from build123d import *

# Parameters (mm, degrees)
F2_DEPTH = 25
F3_DEPTH = 25


with BuildPart() as f2:
    # F1 (on Front) → F2 (new body)
    with BuildSketch(Plane.XZ):
        with BuildLine():
            ThreePointArc((14.696938, -3), (14.924042, -1.507634), (15, 0))
            ThreePointArc((15, 0), (14.924042, 1.507634), (14.696938, 3))
            ThreePointArc((14.696938, 3), (13.858193, 5.740251), (12.513625, 8.270985))
            ThreePointArc((12.513625, 8.270985), (10.606602, 10.606602), (8.270985, 12.513625))
            ThreePointArc((8.270985, 12.513625), (5.740251, 13.858193), (3, 14.696938))
            ThreePointArc((3, 14.696938), (0, 15), (-3, 14.696938))
            ThreePointArc((-3, 14.696938), (-5.740251, 13.858193), (-8.270985, 12.513625))
            ThreePointArc((-8.270985, 12.513625), (-10.606602, 10.606602), (-12.513625, 8.270985))
            ThreePointArc((-12.513625, 8.270985), (-13.858193, 5.740251), (-14.696938, 3))
            ThreePointArc((-14.696938, 3), (-15, 0), (-14.696938, -3))
            ThreePointArc((-14.696938, -3), (-13.858193, -5.740251), (-12.513625, -8.270985))
            ThreePointArc((-12.513625, -8.270985), (-10.606602, -10.606602), (-8.270985, -12.513625))
            ThreePointArc((-8.270985, -12.513625), (-5.740251, -13.858193), (-3, -14.696938))
            ThreePointArc((-3, -14.696938), (0, -15), (3, -14.696938))
            ThreePointArc((3, -14.696938), (5.740251, -13.858193), (8.270985, -12.513625))
            ThreePointArc((8.270985, -12.513625), (10.606602, -10.606602), (12.513625, -8.270985))
            ThreePointArc((12.513625, -8.270985), (13.858193, -5.740251), (14.696938, -3))
        make_face()
        with BuildLine():
            ThreePointArc((-12.513625, 8.270985), (-10.606602, 10.606602), (-8.270985, 12.513625))
            Line((-8.270985, 12.513625), (-11.860811, 16.103452))
            ThreePointArc((-11.860811, 16.103452), (-14.142136, 14.142136), (-16.103452, 11.860811))
            Line((-16.103452, 11.860811), (-12.513625, 8.270985))
        make_face()
        with BuildLine():
            ThreePointArc((-14.696938, -3), (-15, 0), (-14.696938, 3))
            Line((-14.696938, 3), (-19.77372, 3))
            ThreePointArc((-19.77372, 3), (-20, 0), (-19.77372, -3))
            Line((-19.77372, -3), (-14.696938, -3))
        make_face()
        with BuildLine():
            Line((-11.860811, -16.103452), (-8.270985, -12.513625))
            ThreePointArc((-8.270985, -12.513625), (-10.606602, -10.606602), (-12.513625, -8.270985))
            Line((-12.513625, -8.270985), (-16.103452, -11.860811))
            ThreePointArc((-16.103452, -11.860811), (-14.142136, -14.142136), (-11.860811, -16.103452))
        make_face()
        with BuildLine():
            Line((3, -19.77372), (3, -14.696938))
            ThreePointArc((3, -14.696938), (0, -15), (-3, -14.696938))
            Line((-3, -14.696938), (-3, -19.77372))
            ThreePointArc((-3, -19.77372), (0, -20), (3, -19.77372))
        make_face()
        with BuildLine():
            Line((16.103452, -11.860811), (12.513625, -8.270985))
            ThreePointArc((12.513625, -8.270985), (10.606602, -10.606602), (8.270985, -12.513625))
            Line((8.270985, -12.513625), (11.860811, -16.103452))
            ThreePointArc((11.860811, -16.103452), (14.142136, -14.142136), (16.103452, -11.860811))
        make_face()
        with BuildLine():
            ThreePointArc((14.696938, 3), (14.924042, 1.507634), (15, 0))
            ThreePointArc((15, 0), (14.924042, -1.507634), (14.696938, -3))
            Line((14.696938, -3), (19.77372, -3))
            ThreePointArc((19.77372, -3), (20, 0), (19.77372, 3))
            Line((19.77372, 3), (14.696938, 3))
        make_face()
        with BuildLine():
            ThreePointArc((8.270985, 12.513625), (10.606602, 10.606602), (12.513625, 8.270985))
            Line((12.513625, 8.270985), (16.103452, 11.860811))
            ThreePointArc((16.103452, 11.860811), (14.142136, 14.142136), (11.860811, 16.103452))
            Line((11.860811, 16.103452), (8.270985, 12.513625))
        make_face()
        with BuildLine():
            ThreePointArc((-3, 14.696938), (0, 15), (3, 14.696938))
            Line((3, 14.696938), (3, 19.77372))
            ThreePointArc((3, 19.77372), (0, 20), (-3, 19.77372))
            Line((-3, 19.77372), (-3, 14.696938))
        make_face()
    extrude(amount=F2_DEPTH)

    # F0 (on Front) → F3 (cut)
    with BuildSketch(Plane.XZ):
        with BuildLine():
            Line((-5.338161, 7.245967), (-4.582543, 5.937197))
            ThreePointArc((-4.582543, 5.937197), (-5.303301, 5.303301), (-5.937197, 4.582543))
            Line((-5.937197, 4.582543), (-7.245967, 5.338161))
            ThreePointArc((-7.245967, 5.338161), (-7.794229, 4.5), (-8.245967, 3.606111))
            Line((-8.245967, 3.606111), (-6.937197, 2.850492))
            ThreePointArc((-6.937197, 2.850492), (-7.244444, 1.941143), (-7.433034, 1))
            Line((-7.433034, 1), (-8.944272, 1))
            ThreePointArc((-8.944272, 1), (-9, 0), (-8.944272, -1))
            Line((-8.944272, -1), (-7.433034, -1))
            ThreePointArc((-7.433034, -1), (-7.244444, -1.941143), (-6.937197, -2.850492))
            Line((-6.937197, -2.850492), (-8.245967, -3.606111))
            ThreePointArc((-8.245967, -3.606111), (-7.794229, -4.5), (-7.245967, -5.338161))
            Line((-7.245967, -5.338161), (-5.937197, -4.582543))
            ThreePointArc((-5.937197, -4.582543), (-5.303301, -5.303301), (-4.582543, -5.937197))
            Line((-4.582543, -5.937197), (-5.338161, -7.245967))
            ThreePointArc((-5.338161, -7.245967), (-4.5, -7.794229), (-3.606111, -8.245967))
            Line((-3.606111, -8.245967), (-2.850492, -6.937197))
            ThreePointArc((-2.850492, -6.937197), (-1.941143, -7.244444), (-1, -7.433034))
            Line((-1, -7.433034), (-1, -8.944272))
            ThreePointArc((-1, -8.944272), (0, -9), (1, -8.944272))
            Line((1, -8.944272), (1, -7.433034))
            ThreePointArc((1, -7.433034), (1.941143, -7.244444), (2.850492, -6.937197))
            Line((2.850492, -6.937197), (3.606111, -8.245967))
            ThreePointArc((3.606111, -8.245967), (4.5, -7.794229), (5.338161, -7.245967))
            Line((5.338161, -7.245967), (4.582543, -5.937197))
            ThreePointArc((4.582543, -5.937197), (5.303301, -5.303301), (5.937197, -4.582543))
            Line((5.937197, -4.582543), (7.245967, -5.338161))
            ThreePointArc((7.245967, -5.338161), (7.794229, -4.5), (8.245967, -3.606111))
            Line((8.245967, -3.606111), (6.937197, -2.850492))
            ThreePointArc((6.937197, -2.850492), (7.244444, -1.941143), (7.433034, -1))
            Line((7.433034, -1), (8.944272, -1))
            ThreePointArc((8.944272, -1), (9, 0), (8.944272, 1))
            Line((8.944272, 1), (7.433034, 1))
            ThreePointArc((7.433034, 1), (7.244444, 1.941143), (6.937197, 2.850492))
            Line((6.937197, 2.850492), (8.245967, 3.606111))
            ThreePointArc((8.245967, 3.606111), (7.794229, 4.5), (7.245967, 5.338161))
            Line((7.245967, 5.338161), (5.937197, 4.582543))
            ThreePointArc((5.937197, 4.582543), (5.303301, 5.303301), (4.582543, 5.937197))
            Line((4.582543, 5.937197), (5.338161, 7.245967))
            ThreePointArc((5.338161, 7.245967), (4.5, 7.794229), (3.606111, 8.245967))
            Line((3.606111, 8.245967), (2.850492, 6.937197))
            ThreePointArc((2.850492, 6.937197), (1.941143, 7.244444), (1, 7.433034))
            Line((1, 7.433034), (1, 8.944272))
            ThreePointArc((1, 8.944272), (0, 9), (-1, 8.944272))
            Line((-1, 8.944272), (-1, 7.433034))
            ThreePointArc((-1, 7.433034), (-1.941143, 7.244444), (-2.850492, 6.937197))
            Line((-2.850492, 6.937197), (-3.606111, 8.245967))
            ThreePointArc((-3.606111, 8.245967), (-4.5, 7.794229), (-5.338161, 7.245967))
        make_face()
    extrude(amount=F3_DEPTH, mode=Mode.SUBTRACT)


solid = f2.part
Could you check a few things on this model? Use its own coordinates, in mm. A direction names the side the tool comes from. Round coordinates to 2 decimals unless told otherwise and drop trailing zeros. Loops run counter-clockwise (first coordinate to the right, second up) from the corner with the lowest first, then second, coordinate; pieces in that order, holes last. Notation, with made-up numbers: (50, -34.75) - (62, -34.75) arc R28 ccw to (62, -10.75) - close; hole circle Ø8 at (-7, 5). An arc over 180 degrees is marked (long way). Write item = value, one per line.
1) Imagine slicing it at A-A (z = -2). Please give me the cut outline in (x, y), and give its area (3 significant figures).
Computed:
outline = (-19.9, -25) - (-7.23, -25) - (-7.23, 0) - (-19.9, 0) - close; (7.23, -25) - (19.9, -25) - (19.9, 0) - (7.23, 0) - close
area = 634 mm2
2) I'm going to push flat-ended pins straight in: P1, Ø3, axis at y = -5.5, z = 12.5, coming from the -X side; P2, Ø5.5, axis at y = -7, z = 18.5, coming from the +X side; P3, Ø1.5, axis at y = -4, z = -11, coming from the +X side. Where does each tip first touch, or does it pass through?
Computed:
P1 = -16.1
P2 = 12.33
P3 = 15.99
3) I need wall thicknesses on line 1 along Z through (x, y) = (-16, -7.25); line 2 along Z through (x, y) = (5, -9); line 3 along Z through (x, y) = (13, -22). Which ranges of each line are inside material? Lowest first, please. Write a range as from..to.
Computed:
line_1 = -12..-11.76, -3..3, 11.76..12
line_2 = -14.14..-7.48, -6.66..-5.59, 5.59..6.66, 7.48..14.14
line_3 = -15.2..-8.76, -7.48..7.48, 8.76..15.2
4) Imagine slicing it at C-C (z = -13.5). Please give me the cut outline in (x, y).
Computed:
outline = (-14.76, -25) - (-9.26, -25) - (-9.26, 0) - (-14.76, 0) - close; (-6.54, -25) - (6.54, -25) - (6.54, 0) - (-6.54, 0) - close; (9.26, -25) - (14.76, -25) - (14.76, 0) - (9.26, 0) - close
5) Imagine slicing it at B-B (x = -1.5). Please give me the cut outline in (y, z).
Computed:
outline = (-25, -19.94) - (0, -19.94) - (0, -7.35) - (-25, -7.35) - close; (-25, 7.35) - (0, 7.35) - (0, 19.94) - (-25, 19.94) - close
6) Imagine slicing it at D-D (x = 9.5). Please give me the cut outline in (y, z), and give its area (3 significant figures).
Computed:
outline = (-25, -13.74) - (0, -13.74) - (0, 13.74) - (-25, 13.74) - close
area = 687 mm2
7) If we mould it in two halves opening along X, with no side actions, what happens to faces 1 (the flat face through (14.33, -12.32, -10.09)), 2 (the flat face through (10.09, -12.32, 14.33)), 3 (the flat face through (-14.33, -12.32, 10.09)), 4 (the flat face through (17, -12, 3))? For each: pulls with the +X half, pulls with the -X half, needs draft (parallel to the pull), parting line crosses it, or undercut.
Computed:
face_1 = pulls with the +X half
face_2 = undercut
face_3 = pulls with the -X half
face_4 = needs draft
8) On a 3-axis mill with a long thin cutter (end or side, diameter ignored), from which of +Z, -Z, +X, -X, +Y, -Y can I reach the whole of each face in a straight line? I mean faces 5 (the flat face through (-14.28, -12.32, -10.04)), 6 (the cylindrical face through (-5.703, -12.325, 13.874)), 7 (the flat face through (17, -12, -3)), 8 (the flat face through (-1, -12, -8)). Say none if no direction works.
Computed:
face_5 = -X, +Y, -Y
face_6 = +Z, +Y, -Y
face_7 = +X, +Y, -Y
face_8 = +Y, -Y
